```python
from build123d import *

# Parameters (mm, degrees)
SKETCH1_W                         = 128.016
SKETCH1_H                         = 38.1
MAIN_BODY_DEPTH                   = 3.175
SKETCH2_R                         = 1.397
UBRACKET_HOLES_DEPTH              = 4.175
SKETCH3_W                         = 3.175
SKETCH3_H                         = 6.35
TABS_DEPTH                        = 3.175
SKETCH4_RX                        = 11.43
SKETCH4_RY                        = 5.08
SKETCH4_RX_2                      = 10.16
SKETCH4_RY_2                      = 5.842
SKETCH4_RX_3                      = 6.858
SKETCH4_RY_3                      = 5.588
HOLES_FOR_CONTROL_ARMS_DEPTH      = 4.175
SKETCH5_W                         = 3.175
SKETCH5_H                         = 19.05
SLOT_FOR_NOSE_PANEL_DEPTH         = 4.1750001
CUT_CORNER_FOR_SCREW_ACCESS_DEPTH = 4.1750001


with BuildPart() as part:
    # Sketch1 → main body (new body)
    with BuildSketch(Plane.XY):
        Rectangle(SKETCH1_W, SKETCH1_H)
    extrude(amount=MAIN_BODY_DEPTH)

    # Sketch2 → ubracket holes (cut, through all)
    with BuildSketch(Plane.XY.offset(3.175)):
        with Locations((-29.718, -0.508)):
            Circle(SKETCH2_R)
        with Locations((-37.338, -0.508)):
            Circle(SKETCH2_R)
    ubracket_holes = extrude(amount=-UBRACKET_HOLES_DEPTH, mode=Mode.SUBTRACT)

    # Sketch3 → tabs (add)
    with BuildSketch(Plane.XY.offset(3.175)):
        with Locations((-65.5955, 10.795)):
            Rectangle(SKETCH3_W, SKETCH3_H)
        with Locations((-65.5955, -5.715)):
            Rectangle(SKETCH3_W, SKETCH3_H)
        Polygon((-33.528, -19.05), (-30.353, -19.05), (-30.353, -22.2758), (-36.703, -22.2758), (-36.703, -19.05), align=None)
    tabs = extrude(amount=-TABS_DEPTH)

    # Sketch4 → holes for control arms (cut, through all)
    with BuildSketch(Plane.XY.offset(3.175)):
        with Locations(Location((-14.478, 2.54), (0, 0, 90))):
            Ellipse(SKETCH4_RX, SKETCH4_RY)
        with Locations((-33.527531332, -10.668)):
            Ellipse(SKETCH4_RX_2, SKETCH4_RY_2)
        with Locations(Location((-47.498, -1.27), (0, 0, 90))):
            Ellipse(SKETCH4_RX_3, SKETCH4_RY_3)
    holes_for_control_arms = extrude(amount=-HOLES_FOR_CONTROL_ARMS_DEPTH, mode=Mode.SUBTRACT)

    # mirror of ubracket holes: ubracket holes across plane
    add(ubracket_holes.mirror(Plane(origin=(0, 0, 0), x_dir=(0, 0, 1), z_dir=(1, 0, 0))), mode=Mode.SUBTRACT)

    # mirror of tabs: tabs across plane
    add(tabs.mirror(Plane(origin=(0, 0, 0), x_dir=(0, 0, 1), z_dir=(1, 0, 0))))

    # Mirror3: holes for control arms across plane
    add(holes_for_control_arms.mirror(Plane(origin=(0, 0, 0), x_dir=(0, 0, 1), z_dir=(1, 0, 0))), mode=Mode.SUBTRACT)

    # Sketch5 → slot for nose panel (cut, through all)
    with BuildSketch(Plane.XY.offset(3.175)):
        with Locations((0.130633012, -9.525)):
            Rectangle(SKETCH5_W, SKETCH5_H)
    extrude(amount=-SLOT_FOR_NOSE_PANEL_DEPTH, mode=Mode.SUBTRACT)

    # Sketch6 → cut corner for screw access (cut, through all)
    with BuildSketch(Plane.XY.offset(3.175)):
        with BuildLine():
            Line((0, -19.05), (0, -11.43))
            ThreePointArc((0, -11.43), (-7.135959689, -13.930067184), (-12.7, -19.05))
            Line((-12.7, -19.05), (0, -19.05))
        make_face()
        with BuildLine():
            Line((-64.008, -19.05), (-55.118, -19.05))
            ThreePointArc((-55.118, -19.05), (-57.721820715, -12.763820715), (-64.008, -10.16))
            Line((-64.008, -10.16), (-64.008, -19.05))
        make_face()
    cut_corner_for_screw_access = extrude(amount=-CUT_CORNER_FOR_SCREW_ACCESS_DEPTH, mode=Mode.SUBTRACT)

    # Mirror4: cut corner for screw access across plane
    add(cut_corner_for_screw_access.mirror(Plane(origin=(0, 0, 0), x_dir=(0, 0, 1), z_dir=(1, 0, 0))), mode=Mode.SUBTRACT)


solid = part.part
```
Design review of the part built by this model. Coordinates are the model's own, in mm. A direction names the side the tool comes from. Give positions to 0.01 mm unless a question says otherwise; leave off trailing zeros. One line per item, written item: value.
Q1. We need section A-A on z = 0.5. Give the number of separate pieces and of enclosed holes in the cut face, and give its area (3 significant figures).
Numbers:
separate pieces: 1
enclosed holes: 10
area: 3,710 mm^2
Q2. For L1, parallel to X at y = 10, z = 1.1; L2, parallel to X at y = 8, z = 2.55; L3, parallel to Y at x = -42.5, z = 1.6, list the stretches that pass through material, from the lowest coordinate up.
Numbers:
L1: x = -67.18 to -18.33, -10.63 to 10.63, 18.33 to 67.18
L2: x = -67.18 to -18.94, -10.02 to 10.02, 18.94 to 67.18
L3: y = -19.05 to -13.41, -7.93 to -4.34, 1.8 to 19.05
Q3. For pin 1 Ø1.6 at (x, z) = (-25, 1) entering from -Y; pin 2 Ø1.6 at (x, z) = (-65, 2) entering from +Y; pin 3 Ø0.6 at (y, z) = (-9.5, 1) entering from +X, all flat-tipped, find the tip position at first contact; note any pin that passes through.
Numbers:
pin 1: stops at y = -19.05
pin 2: stops at y = 13.97
pin 3: stops at x = 64.01
Q4. Draft analysis for pull direction X (two halves, no side actions). For faces 1 (the cylindrical face through (-31.114, -0.447, 1.61)), 2 (the flat face through (-64.008, 2, 2)), 3 (the flat face through (-66, -8.89, 2)), 4 (the cylindrical face through (-36.048, -1.043, 1.61)), state which applies: pulls with the +X half, pulls with the -X half, needs draft (parallel to the pull), parting line crosses it, or undercut.
Numbers:
face 1: undercut
face 2: pulls with the -X half
face 3: needs draft
face 4: undercut
Q5. Machinability: for faces 5 (the flat face through (-64.008, 16, 2)), 6 (the flat face through (66, 7.62, 2)), 7 (the flat face through (-22, -19.05, 2)), 8 (the flat face through (-66, 7.62, 2)), 9 (the flat face through (64.008, 16, 2)), which of the approach directions +Z, -Z, +X, -X, +Y, -Y give a long, thin tool a straight path to every point of the face, cutting with its end or side? Answer none if there is none.
Numbers:
face 5: +Z, -Z, -X, +Y
face 6: +Z, -Z, +X
face 7: +Z, -Z, -Y
face 8: +Z, -Z, -X
face 9: +Z, -Z, +X, +Y
